from build123d import *

# Parameters (mm, degrees)
SKETCH001_R     = 45
PAD_DEPTH       = 1
SKETCH_W        = 8
SKETCH_H        = 70
PAD003_DEPTH    = 3
FILLET_R        = 0.6
PAD006_DEPTH    = 6
SKETCH015_R     = 1.4
POCKET008_DEPTH = 15
FILLET008_R     = 1


with BuildPart() as part:
    # Sketch001 → Pad (new body)
    with BuildSketch(Plane.XY):
        with BuildLine():
            Line((60, 64), (0, 64))
            ThreePointArc((0, 64), (-63.999918, 0), (0, -64))
            Line((60, -64), (0, -64))
            ThreePointArc((60, -64), (69.192388, -60.192388), (73, -51))
            Line((73, 51), (73, -51))
            ThreePointArc((73, 51), (69.192388, 60.192388), (60, 64))
        make_face()
        Circle(SKETCH001_R, mode=Mode.SUBTRACT)
    extrude(amount=-PAD_DEPTH)

    # Sketch → Pad003 (new body)
    with BuildSketch(Plane.XY):
        with Locations((69, 0)):
            Rectangle(SKETCH_W, SKETCH_H)
    extrude(amount=PAD003_DEPTH)

    # Fillet
    fillet_edges = [part.edges().sort_by_distance(p)[0] for p in [
        (69.192388, 60.192388, -1),
        (30, 64, -1),
        (-63.999918, 0, -1),
        (30, -64, -1),
        (69.192388, -60.192388, -1),
        (73, 0, -1),
        (-45, 0, -1),
    ]]
    fillet(fillet_edges, radius=FILLET_R)

    # Sketch014 → Pad006 (new body)
    with BuildSketch(Plane.YZ.offset(73)):
        with BuildLine():
            Line((-35, 3), (-24.5, 31))
            Line((-24.5, 31), (-18.2, 31))
            ThreePointArc((-18.2, 31), (-7, 19.8), (4.2, 31))
            Line((4.2, 31), (10.5, 31))
            Line((10.5, 31), (35, 3))
            Line((35, 3), (-35, 3))
        make_face()
    extrude(amount=-PAD006_DEPTH)

    # Sketch015 → Pocket008 (cut)
    with BuildSketch(Plane.XY.offset(31)):
        with Locations((70, 7)):
            Circle(SKETCH015_R)
        with Locations((70, -21)):
            Circle(SKETCH015_R)
    extrude(amount=-POCKET008_DEPTH, mode=Mode.SUBTRACT)

    # Fillet008
    fillet008_edges = [part.edges().sort_by_distance(p)[0] for p in [
        (73, 22.75, 17),
        (67, 22.75, 17),
        (67, -29.75, 17),
        (73, -29.75, 17),
    ]]
    fillet(fillet008_edges, radius=FILLET008_R)


solid = part.part
Part model, mm, in its own coordinate system. A direction names the side the tool comes from. Coordinates: 2 decimals unless noted, no trailing zeros. Order: outer loops, then holes, each group sorted by start corner. A loop starts at its lowest first (then second) coordinate and runs counter-clockwise, first axis right, second up. Notation, with made-up numbers: M 71.5,-21 L 106.5,-21 A22 cw 106.5,0 Z; hole C -2.5,51.25 d7. An arc over 180 degrees is marked long. One line per question, with ' | ' between items.
Q1. Pin check, flat tips, straight feed: P1, Ø0.9, axis at x = 66.5, y = 0.5, coming from the +Z side; P2, Ø14, axis at y = -16.5, z = 16, coming from the -X side; P3, Ø2.5, axis at x = 67.5, z = 1.5, coming from the +Y side. Stop position of each tip, or through.
A:
P1: stops at z = 3 | P2: stops at x = 67 | P3: stops at y = 35
Q2. Slice it at A-A (z = 24). Count the separate pieces of the cut face and the enclosed holes in it, and give its area (3 significant figures).
A:
separate pieces: 2 | enclosed holes: 2 | area: 144 mm^2
Q3. 3-axis set-ups, long thin cutter, end or side, ignore diameter. For faces 1 (the face through (69.091, -60.293, -0.197)), 2 (the face through (67, 0, 14)): which of +Z, -Z, +X, -X, +Y, -Y reach the whole face in a straight line?
A:
face 1: +Z, -Z, +X, -Y | face 2: +Z, -X, +Y, -Y
Q4. Slice it at B-B (y = 0). Give the cut face in (x, z), and give its area (3 significant figures).
A:
outline: M -64,-0.4 A0.6 ccw -63.4,-1 L -45.6,-1 A0.6 ccw -45,-0.4 L -45,0 L -64,0 Z; M 45,-0.4 A0.6 ccw 45.6,-1 L 72.4,-1 A0.6 ccw 73,-0.4 L 73,22.26 L 67,22.26 L 67,3 L 65,3 L 65,0 L 45,0 Z | area: 186 mm^2
Q5. Two-plate mould, pull along Y, no slides. Class faces 3 (the face through (70.028, -29.824, 16.804)), 4 (the face through (70, -7.2, 19.8)), 5 (the face through (49, 1, 0)): +Y half, -Y half, draft (parallel to the pull), parting line (faces both ways), or undercut.
A:
face 3: -Y half | face 4: undercut | face 5: draft
Q6. Drill centre lines: line 1 (Y direction, x = 70, z = 25); line 2 (Y direction, x = 70, z = 22.5); line 3 (Y direction, x = 70, z = 19). Where is each one in solid material? Low to high.
A:
line 1: y = -26.75 to -22.4, -19.6 to -16.46, 2.46 to 5.6, 8.4 to 15.75 | line 2: y = -27.69 to -22.4, -19.6 to -14.29, 0.29 to 5.6, 8.4 to 17.94 | line 3: y = -29 to -22.4, -19.6 to 5.6, 8.4 to 21
